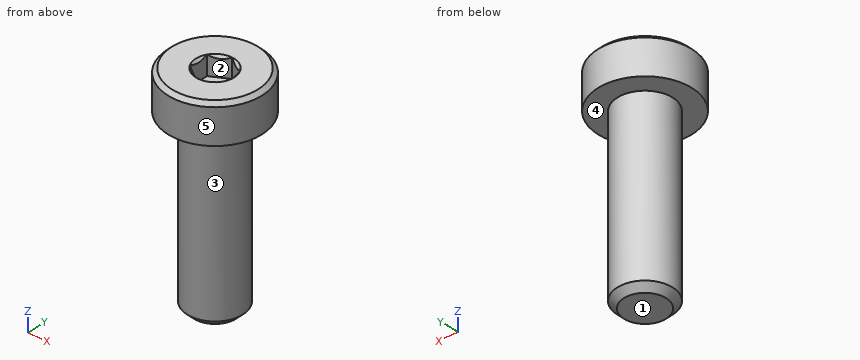
```python
from build123d import *

# Parameters (mm, degrees)
CUT_EXTRUDE1_DEPTH = 1.75


with BuildPart() as part:
    # Sketch2 → Revolve1 (revolve)
    with BuildSketch(Plane(origin=(0, 0, 0), x_dir=(0, 0, -1), z_dir=(1, 0, 0)), mode=Mode.PRIVATE) as revolve1_sk:
        Polygon((-9.75, 0), (-9.75, 3.9), (-9.4, 4.25), (-6.25, 4.25), (-6.25, 2.5), (9.15, 2.5), (9.75, 1.9), (9.75, 0), align=None)
    revolve(revolve1_sk.sketch.rotate(Axis((0, 0, -9.75), (0, 0, 1)), 90), axis=Axis((0, 0, -9.75), (0, 0, 1)))

    # Sketch4 → Cut-Extrude1 (cut)
    with BuildSketch(Plane.XY.offset(9.75)):
        Polygon((1.5, -0.866025404), (1.5, 0.866025404), (0, 1.732050808), (-1.5, 0.866025404), (-1.5, -0.866025404), (0, -1.732050808), align=None)
    extrude(amount=-CUT_EXTRUDE1_DEPTH, mode=Mode.SUBTRACT)

    # Cut-Extrude2 cone 1 section (through the dimple's axis) → Cut-Extrude2 (revolve, cut)
    with BuildSketch(Plane(origin=(0, 0, 9.75), x_dir=(0, -1, 0), z_dir=(1, 0, 0))):
        Polygon((0, 0), (1.732050808, 0), (0, 1.732050808), align=None)
    revolve(axis=Axis((0, 0, 9.75), (0, 0, -1)), mode=Mode.SUBTRACT)


solid = part.part
```
Build history of the part. All positions in model axes, mm. Face numbers are marked on the shaded views. A direction names the side the tool comes from. Round coordinates to 2 decimals unless told otherwise and drop trailing zeros. Order: outer loops, then holes, each group sorted by start corner. A loop starts at its lowest first (then second) coordinate and runs counter-clockwise, first axis right, second up. Notation, with made-up numbers: (12.5, 2) -> (46.5, 2) arc R10 ccw to (46.5, 17) -> close; hole circle Ø5 at (-9, 59). An arc over 180 degrees is marked (long way). Answer in a Markdown table with one row per item.
1) Which spindle directions (+Z, -Z, +X, -X, +Y, -Y) get a long thin tool onto all of the face, cutting with end or side? Do the marked faces 4 and 5. Say none if no direction does.
Values:
| item | result |
|---|---|
| face 4 | -Z |
| face 5 | +Z, -Z |
2) Band-saw the part on A-A on y = 0. Give the cut face in (x, z).
Values:
| item | result |
|---|---|
| outline | (-4.25, 6.25) -> (-2.5, 6.25) -> (-2.5, -9.15) -> (-1.9, -9.75) -> (1.9, -9.75) -> (2.5, -9.15) -> (2.5, 6.25) -> (4.25, 6.25) -> (4.25, 9.4) -> (3.9, 9.75) -> (1.73, 9.75) -> (1.5, 9.52) -> (1.5, 8) -> (-1.5, 8) -> (-1.5, 9.52) -> (-1.73, 9.75) -> (-3.9, 9.75) -> (-4.25, 9.4) -> close |
3) Pin check, flat tips, straight feed: P1, Ø2, axis at y = -3, z = -3, coming from the -X side; P2, Ø5, axis at x = 3, z = -5, coming from the +Y side; P3, Ø2, axis at x = -0.5, z = 0, coming from the -Y side. Stop position of each tip, or through.
Values:
| item | result |
|---|---|
| P1 | x = -1.5 |
| P2 | y = 2.45 |
| P3 | y = -2.5 |
4) Band-saw the part on B-B on z = -5.5. Give the cut face in (x, y).
Values:
| item | result |
|---|---|
| outline | circle Ø5 at (0, 0) |
5) Wall check: L1, parallel to Z at x = -1, y = 3.25; L2, parallel to Y at x = -2, z = 5.5. Give the ranges that are in metal, low to high.
Values:
| item | result |
|---|---|
| L1 | 6.25 to 9.75 |
| L2 | -1.5 to 1.5 |
6) Mould opens along X. For the marked faces 1, 2 and 3 say: released by +X, released by -X, zero draft, split by the parting line, or undercut.
Values:
| item | result |
|---|---|
| face 1 | zero draft |
| face 2 | undercut |
| face 3 | split by the parting line |
